from build123d import *

# Parameters (mm, degrees)
F0_W     = 76.2
F0_H     = 25.4
F1_DEPTH = 152.4
F2_W     = 25.4
F2_H     = 127
F3_DEPTH = 25.4
F5_DEPTH = 25.4


with BuildPart() as f1:
    # F0 (on Front) → F1 (new body)
    with BuildSketch(Plane.XZ):
        with Locations((38.1, 12.7)):
            Rectangle(F0_W, F0_H)
    extrude(amount=-F1_DEPTH)

    # F2 (on face) → F3 (join)
    with BuildSketch(Plane.XY.offset(25.4)):
        Polygon((0, 25.4), (0, 0), (76.2, 0), (76.2, 25.4), (50.8, 25.4), (25.4, 25.4), align=None)
        with Locations((38.1, 88.9)):
            Rectangle(F2_W, F2_H)
    extrude(amount=F3_DEPTH)

    # F4 (on face) → F5 (cut)
    with BuildSketch(Plane.YZ.offset(50.8)):
        Polygon((152.4, 50.8), (25.4, 50.8), (152.4, 25.4), align=None)
    extrude(amount=-F5_DEPTH, mode=Mode.SUBTRACT)


solid = f1.part
Geometry check sheet. Reference: the model listing, model coordinates, mm. A direction names the side the tool comes from. Give positions to 0.01 mm unless a question says otherwise; leave off trailing zeros. Loops run counter-clockwise (first coordinate to the right, second up) from the corner with the lowest first, then second, coordinate; pieces in that order, holes last. Notation, with made-up numbers: M -5,-9 L 16,-9 A32 ccw 16,18 Z; hole C 28.25,78 d2. An arc over 180 degrees is marked long. Answer as a JSON object with one key per item and string values. Group by question number.
Item 1: Material ranges on L1, parallel to X at y = 33.5, z = 45; L2, parallel to Z at x = 71.5, y = 120.5, recorded low to high.
Item 2: Gauge pin test, flat ends, axial feed: pin 1 (7.5 mm diameter, centred on x = 58.5, y = 108.5, fed in from +Z); pin 2 (1 mm diameter, centred on y = 56, z = 34, fed in from -X); pin 3 (12.5 mm diameter, centred on x = 9.5, z = 40, fed in from +Y). Record the tip position at first contact, or that the pin passes through.
Item 3: Sectioned sample at B-B on z = 47. Record the boundary of the cut face in (x, y).
Item 4: Sectioned sample at A-A on y = 122. Record the boundary of the cut face in (x, z), plus the area to 3 significant figures.
Item 5: Access from +Z, -Z, +X, -X, +Y, -Y to the whole of each face (thin tool, end or side, straight path). Record for faces 1 (the flat face through (38, 152.4, 13)), 2 (the flat face through (64, 25.4, 38)), 3 (the flat face through (13, 88, 25.4)).
Item 6: Sectioned sample at C-C on x = 42.5. Record the boundary of the cut face in (y, z).
Findings below:
{
 "1": {"L1": "25.4 to 50.8", "L2": "0 to 25.4"},
 "2": {"pin 1": "z = 25.4", "pin 2": "x = 25.4", "pin 3": "y = 25.4"},
 "3": {"outline": "M 0,0 L 76.2,0 L 76.2,25.4 L 50.8,25.4 L 50.8,44.4 L 25.4,44.4 L 25.4,25.4 L 0,25.4 Z"},
 "4": {"outline": "M 0,0 L 76.2,0 L 76.2,25.4 L 50.8,25.4 L 50.8,31.48 L 25.4,31.48 L 25.4,25.4 L 0,25.4 Z", "area": "2,090 mm2"},
 "5": {"face 1": "+Z, -Z, +X, -X, +Y", "face 2": "+Z, +X, +Y", "face 3": "+Z, -X, +Y"},
 "6": {"outline": "M 0,0 L 152.4,0 L 152.4,25.4 L 25.4,50.8 L 0,50.8 Z"}
}
